```python
from build123d import *

# Parameters (mm, degrees)
SKETCH1_W                = 30
SKETCH1_H                = 32
BOSS_EXTRUDE1_DEPTH      = 14
CAVITY1_START            = 44.284378121
CAVITY1_OUTLINE_R        = 3
CAVITY1_DEPTH            = 32
M3_CLEARANCE_HOLE1_D     = 3.2
M3_CLEARANCE_HOLE1_DEPTH = 7
M3_CLEARANCE_HOLE1_TIP   = 0.96137699


# Read off the part's stored shape, not the designer's step: Cavity1
with BuildPart() as part:
    # Sketch1 → Boss-Extrude1 (new body)
    with BuildSketch(Plane(origin=(0, 8, 0), x_dir=(1, 0, 0), z_dir=(0, 1, 0))):
        with Locations((0, -60.284378121)):
            Rectangle(SKETCH1_W, SKETCH1_H)
    extrude(amount=-BOSS_EXTRUDE1_DEPTH)

    # Cavity1 outline → Cavity1 (cut)
    with BuildSketch(Plane.XY.offset(CAVITY1_START)):
        Circle(CAVITY1_OUTLINE_R)
    extrude(amount=CAVITY1_DEPTH, mode=Mode.SUBTRACT)

    # M3 Clearance Hole1
    with Locations(Plane(origin=(0, 8, 0), x_dir=(1, 0, 0), z_dir=(0, 1, 0))):
        with Locations((10.5, -49.784378121), (-10.5, -49.784378121), (-10.5, -70.784378121), (10.5, -70.784378121)):
            Hole(M3_CLEARANCE_HOLE1_D / 2, depth=M3_CLEARANCE_HOLE1_DEPTH)
            with Locations((0, 0, -(M3_CLEARANCE_HOLE1_DEPTH + M3_CLEARANCE_HOLE1_TIP / 2))):  # 118° drill point
                Cone(0, M3_CLEARANCE_HOLE1_D / 2, M3_CLEARANCE_HOLE1_TIP, mode=Mode.SUBTRACT)


solid = part.part
```
Could you check a few things on this model? Use its own coordinates, in mm. A direction names the side the tool comes from. Give positions to 0.01 mm unless a question says otherwise; leave off trailing zeros. Loops run counter-clockwise (first coordinate to the right, second up) from the corner with the lowest first, then second, coordinate; pieces in that order, holes last. Notation, with made-up numbers: (46.25, -12.5) -> (73.25, -12.5) arc R36 ccw to (73.25, 26.5) -> close; hole circle Ø4 at (-27.75, 65.25). An arc over 180 degrees is marked (long way). Put each result on its own line as item: value.
(1) Imagine slicing it at C-C on z = 57. Write out the boundary of the cut face in (x, y).
Computed:
outline: (-15, -6) -> (15, -6) -> (15, 8) -> (-15, 8) -> close; hole circle Ø6 at (0, 0)
(2) Imagine slicing it at D-D on y = 5.75. Write out the boundary of the cut face in (x, z), plus the area to 3 significant figures.
Computed:
outline: (-15, 44.28) -> (15, 44.28) -> (15, 76.28) -> (-15, 76.28) -> close; hole circle Ø3.2 at (-10.5, 49.78); hole circle Ø3.2 at (-10.5, 70.78); hole circle Ø3.2 at (10.5, 49.78); hole circle Ø3.2 at (10.5, 70.78)
area: 928 mm^2
(3) Please list where these lines run through material, in increasing order: probe 1 along Z at (x, y) = (10.5, 6.25); probe 2 along Z at (x, y) = (-11.25, 1.5); probe 3 along Y at (x, z) = (0, 57). Write a range as [from, to].
Computed:
probe 1: [44.28, 48.18], [51.38, 69.18], [72.38, 76.28]
probe 2: [44.28, 48.37], [51.2, 69.37], [72.2, 76.28]
probe 3: [-6, -3], [3, 8]
(4) Imagine slicing it at A-A on x = 0. Write out the boundary of the cut face in (y, z), plus the area to 3 significant figures.
Computed:
outline: (-6, 44.28) -> (-3, 44.28) -> (-3, 76.28) -> (-6, 76.28) -> close; (3, 44.28) -> (8, 44.28) -> (8, 76.28) -> (3, 76.28) -> close
area: 256 mm^2
(5) I'm going to push flat-ended pins straight in: pin 1 Ø5.5 at (x, y) = (0, 0) entering from -Z; pin 2 Ø3 at (x, z) = (10.5, 70.78) entering from +Y. Where does each tip first touch, or does it pass through?
Computed:
pin 1: through
pin 2: y = 0.94
(6) Imagine slicing it at B-B on y = 2.5. Write out the boundary of the cut face in (x, z).
Computed:
outline: (-15, 44.28) -> (-1.66, 44.28) -> (-1.66, 76.28) -> (-15, 76.28) -> close; (1.66, 44.28) -> (15, 44.28) -> (15, 76.28) -> (1.66, 76.28) -> close; hole circle Ø3.2 at (-10.5, 49.78); hole circle Ø3.2 at (-10.5, 70.78); hole circle Ø3.2 at (10.5, 49.78); hole circle Ø3.2 at (10.5, 70.78)
(7) For faces 1 (the face through (-15, 1, 61)), 2 (the face through (-10.153, 4.451, 72.346)), which set-ups out of +Z, -Z, +X, -X, +Y, -Y let a thin tool reach every point of the face, with its end or its side?
Computed:
face 1: +Z, -Z, -X, +Y, -Y
face 2: +Y
(8) Thinking about a two-plate mould opening in X: for faces 3 (the face through (0, 4, 76.284)), 4 (the face through (-9.23, 4.45, 50.76)), 5 (the face through (15, 1, 61)), which applies, pulls with the +X half, pulls with the -X half, needs draft (parallel to the pull), parting line crosses it, or undercut?
Computed:
face 3: needs draft
face 4: undercut
face 5: pulls with the +X half
